Could you check a few things on this drawing? It's one solid part, dimensions in mm from its lowest x, y, z. A direction names the side the tool comes from. Coordinates: 2 decimals unless noted, no trailing zeros. Loops run counter-clockwise (first coordinate to the right, second up) from the corner with the lowest first, then second, coordinate; pieces in that order, holes last. Notation, with made-up numbers: (-1, 55) -> (18, 55) arc R26 cw to (18, 73) -> close; hole circle Ø8 at (-33, 58). An arc over 180 degrees is marked (long way). One line per question, with ' | ' between items.
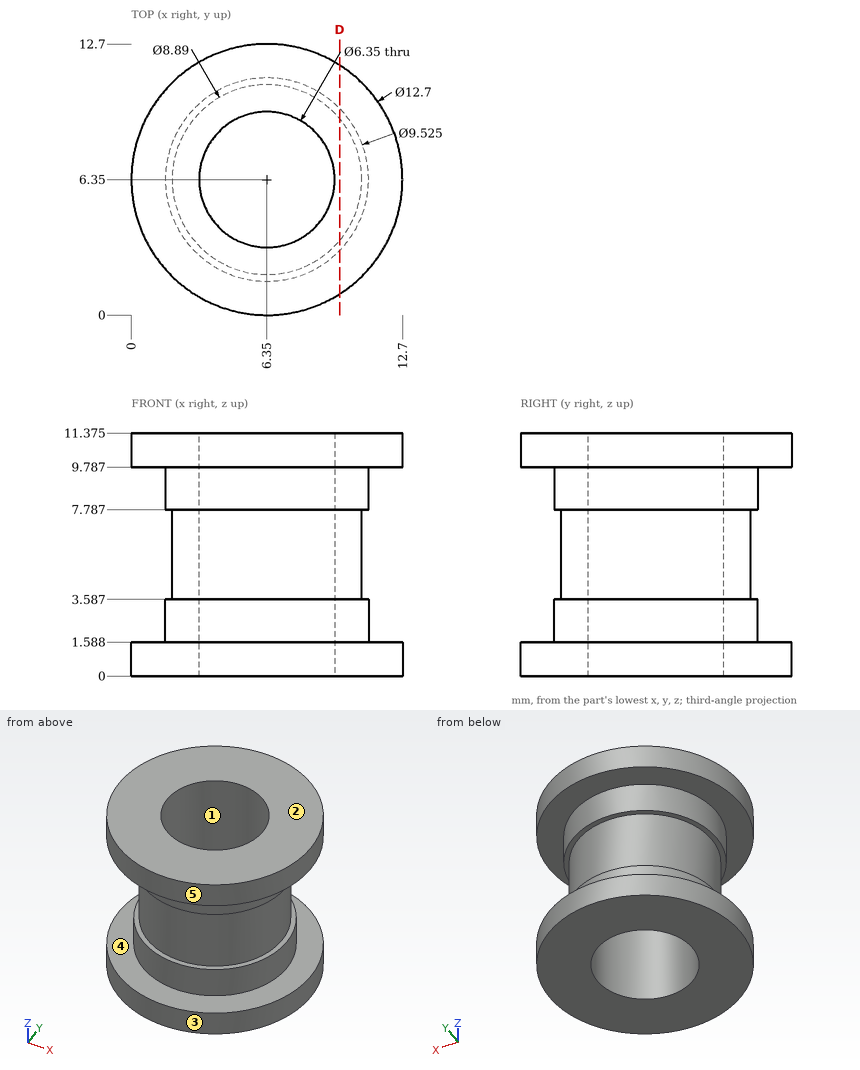
1) If we section it at D-D on x = 9.75: Please give me the cut outline in (y, z) (1 decimal).
Data:
outline: (1, 0) -> (11.7, 0) -> (11.7, 1.6) -> (9.7, 1.6) -> (9.7, 3.6) -> (9.2, 3.6) -> (9.2, 7.8) -> (9.7, 7.8) -> (9.7, 9.8) -> (11.7, 9.8) -> (11.7, 11.4) -> (1, 11.4) -> (1, 9.8) -> (3, 9.8) -> (3, 7.8) -> (3.5, 7.8) -> (3.5, 3.6) -> (3, 3.6) -> (3, 1.6) -> (1, 1.6) -> close
2) I need wall thicknesses on line 1 along Y through (x, z) = (6.35, 9) (1 decimal); line 2 along Z through (x, y) = (9.5, 1) (1 decimal); line 3 along Y through (x, z) = (6.35, 4.25) (1 decimal). Which ranges of each line are inside material? Lowest first, please. Write a range as from..to.
Data:
line 1: 1.6..3.2, 9.5..11.1 | line 2: 0..1.6, 9.8..11.4 | line 3: 1.9..3.2, 9.5..10.8
3) On a 3-axis mill with a long thin cutter (end or side, diameter ignored), from which of +Z, -Z, +X, -X, +Y, -Y can I reach the whole of each face in a straight line? I mean the marked faces 4 and 5. Say none if no direction works.
Data:
face 4: none | face 5: +Z, -Z
4) I'm going to push flat-ended pins straight in: pin 1 Ø6 at (x, z) = (5.5, 6.5) entering from -Y; pin 2 Ø2 at (x, z) = (7.5, 5.5) entering from -Y. Where does each tip first touch, or does it pass through?
Data:
pin 1: y = 1.59 | pin 2: y = 1.91
5) We'd pull the mould along X, two halves only. Please class the marked faces 1, 2 and 3: pulls with the +X half, pulls with the -X half, needs draft (parallel to the pull), parting line crosses it, or undercut.
Data:
face 1: undercut | face 2: needs draft | face 3: parting line crosses it
